```python
from build123d import *

# Parameters (mm, degrees)
SKETCH1_W           = 38
SKETCH1_H           = 70
BOSS_EXTRUDE1_DEPTH = 5
SKETCH2_R           = 1.5
CUT_EXTRUDE1_DEPTH  = 134.018795664
FILLET1_R           = 3
FILLET2_DEPTH       = 5
SKETCH3_W           = 188
SKETCH3_H           = 3
BOSS_EXTRUDE2_DEPTH = 8
SKETCH4_W           = 5
SKETCH4_H           = 39
BOSS_EXTRUDE3_DEPTH = 8
BOSS_EXTRUDE4_DEPTH = 5
FILLET3_SIZE        = 40
FILLET3_SIZE_2      = 10
FILLET4_SIZE        = 40
FILLET4_SIZE_2      = 10
CUT_EXTRUDE2_DEPTH  = 134.165310942


with BuildPart() as part:
    # Sketch1 → Boss-Extrude1 (new body)
    with BuildSketch(Plane.XY):
        with Locations((19, -35)):
            Rectangle(SKETCH1_W, SKETCH1_H)
        Polygon((-75, 15), (-75, 0), (0, 0), (38, 0), (113, 0), (113, 15), align=None)
    extrude(amount=BOSS_EXTRUDE1_DEPTH)

    # Sketch2 → Cut-Extrude1 (cut, through all)
    with BuildSketch(Plane.XY.offset(5)):
        with Locations((34, -66)):
            Circle(SKETCH2_R)
        with Locations((4, -66)):
            Circle(SKETCH2_R)
        with Locations((4, -40)):
            Circle(SKETCH2_R)
        with Locations((34, -40)):
            Circle(SKETCH2_R)
    extrude(amount=-CUT_EXTRUDE1_DEPTH, mode=Mode.SUBTRACT)

    # Fillet1
    fillet1_edges = [part.edges().sort_by_distance(p)[0] for p in [
        (38, -70, 2.5),
        (0, -70, 2.5),
    ]]
    fillet(fillet1_edges, radius=FILLET1_R)

    # Fillet2: read off the stored shape, not the designer's step
    # Fillet2 outline → Fillet2 (add)
    with BuildSketch(Plane.XY):
        with BuildLine():
            add(Edge.make_bspline(
                [(58, 0), (38, 0), (38, -20)],
                knots=[0, 0, 0, 1, 1, 1], degree=2, weights=[1, 0.052631579, 1]))
            Line((58, 0), (38, 0))
            Line((38, 0), (38, -20))
        make_face()
        with BuildLine():
            Line((0, 0), (-20, 0))
            add(Edge.make_bspline(
                [(-20, 0), (0, 0), (0, -20)],
                knots=[0, 0, 0, 1, 1, 1], degree=2, weights=[1, 0.052631579, 1]))
            Line((0, -20), (0, 0))
        make_face()
    extrude(amount=FILLET2_DEPTH)

    # Sketch3 → Boss-Extrude2 (add)
    with BuildSketch(Plane.XY.offset(5)):
        with Locations((19, 4.5)):
            Rectangle(SKETCH3_W, SKETCH3_H)
    extrude(amount=BOSS_EXTRUDE2_DEPTH)

    # Sketch4 → Boss-Extrude3 (add)
    with BuildSketch(Plane.XY.offset(5)):
        with Locations((19, -16.5)):
            Rectangle(SKETCH4_W, SKETCH4_H)
    extrude(amount=BOSS_EXTRUDE3_DEPTH)

    # Sketch5 → Boss-Extrude4 (add)
    with BuildSketch(Plane.XY.offset(5)):
        Polygon((-52, 0), (-57.902965871, 0), (-60, 0), (0, -30), (0, -25), align=None)
        Polygon((38, -30), (98, 0), (90, 0), (38, -25), align=None)
    extrude(amount=-BOSS_EXTRUDE4_DEPTH)

    # Fillet3
    # a fillet whose section is not a circle: 40, 10 mm, written as the material it takes off along each edge
    with BuildSketch(Plane(origin=(-75, 15, -100), x_dir=(1, 0, 0), z_dir=(0, 0, 1))) as fillet3_piece_1:
        with BuildLine():
            Bezier((FILLET3_SIZE, 0), (0, 0), (0, -FILLET3_SIZE_2), weights=[1, 0.707106781, 1])
            Line((0, -FILLET3_SIZE_2), (0, 0))
            Line((0, 0), (FILLET3_SIZE, 0))
        make_face()
    extrude(amount=205, mode=Mode.SUBTRACT)

    # Fillet4
    # a fillet whose section is not a circle: 40, 10 mm, written as the material it takes off along each edge
    with BuildSketch(Plane(origin=(113, 15, -100), x_dir=(-1, 0, 0), z_dir=(0, 0, 1))) as fillet4_piece_1:
        with BuildLine():
            Bezier((FILLET4_SIZE, 0), (0, 0), (0, FILLET4_SIZE_2), weights=[1, 0.707106781, 1])
            Line((0, FILLET4_SIZE_2), (0, 0))
            Line((0, 0), (FILLET4_SIZE, 0))
        make_face()
    extrude(amount=205, mode=Mode.SUBTRACT)

    # Sketch6 → Cut-Extrude2 (cut, through all)
    with BuildSketch(Plane.XY.offset(5)):
        with BuildLine():
            Line((3.671572875, -13.862410437), (-3.399494937, -6.791342626))
            ThreePointArc((-3.399494937, -6.791342626), (-3.399494937, -1.134488376), (2.257359313, -1.134488376))
            Line((2.257359313, -1.134488376), (9.328427125, -8.205556188))
            ThreePointArc((9.328427125, -8.205556188), (9.328427125, -13.862410437), (3.671572875, -13.862410437))
        make_face()
        with BuildLine():
            Line((28.671572875, -8.445013015), (35.742640687, -1.373945203))
            ThreePointArc((35.742640687, -1.373945203), (41.399494937, -1.373945203), (41.399494937, -7.030799453))
            Line((41.399494937, -7.030799453), (34.328427125, -14.101867265))
            ThreePointArc((34.328427125, -14.101867265), (28.671572875, -14.101867265), (28.671572875, -8.445013015))
        make_face()
    extrude(amount=-CUT_EXTRUDE2_DEPTH, mode=Mode.SUBTRACT)


solid = part.part
```
Verification items for the finished model (mm, model axes). A direction names the side the tool comes from. Give positions to 0.01 mm unless a question says otherwise; leave off trailing zeros. Order: outer loops, then holes, each group sorted by start corner. A loop starts at its lowest first (then second) coordinate and runs counter-clockwise, first axis right, second up. Notation, with made-up numbers: (4, -35.5) -> (44, -35.5) arc R27 ccw to (44, -18.5) -> close; hole circle Ø3 at (77.5, -38.75). An arc over 180 degrees is marked (long way). Use a Markdown table: item, result.
1) Material ranges on probe 1 along X at (y, z) = (-66, 3.15); probe 2 along Y at (x, z) = (34, 2.3); probe 3 along X at (y, z) = (-18.5, 3.5), recorded low to high.
Results:
| item | result |
|---|---|
| probe 1 | 0 to 2.5, 5.5 to 32.5, 35.5 to 38 |
| probe 2 | -70 to -67.5, -64.5 to -41.5, -38.5 to -14.4, -3.12 to 15 |
| probe 3 | -23 to -13.52, -1.04 to 39.04, 51.52 to 61 |
2) Depth check by flat-ended pin: pin 1 Ø4 at (y, z) = (-20.5, 9) entering from -X; pin 2 Ø1.5 at (y, z) = (-22, 1.5) entering from +X; pin 3 Ø2 at (y, z) = (-13.5, 4.5) entering from -X; pin 4 Ø1.8 at (x, y) = (4, -40) entering from +Z. Enter the tip coordinate at first touch or a pass-through.
Results:
| item | result |
|---|---|
| pin 1 | x = 16.5 |
| pin 2 | x = 55.5 |
| pin 3 | x = -35 |
| pin 4 | through |
3) Section check C-C, the plane y = -11.5. Give the number of separate pieces and of enclosed holes in the cut face, then the cut area to 3 significant figures.
Results:
| item | result |
|---|---|
| separate pieces | 5 |
| enclosed holes | 0 |
| area | 301 mm² |
4) Section check B-B, the plane x = 13.5. Record the boundary of the cut face in (y, z).
Results:
| item | result |
|---|---|
| outline | (-70, 0) -> (15, 0) -> (15, 5) -> (6, 5) -> (6, 13) -> (3, 13) -> (3, 5) -> (-70, 5) -> close |
5) Tool access check on faces 1 (the flat face through (105, 0, 2)), 2 (the flat face through (-30, 3, 9)), 3 (the flat face through (0.19, -10.38, 2.54)), 4 (the flat face through (21.5, -17, 9)). Record the directions out of +Z, -Z, +X, -X, +Y, -Y that give a thin tool (end or side, any length) a straight path to the whole face; none if there is none.
Results:
| item | result |
|---|---|
| face 1 | +Z, -Z, +X, -Y |
| face 2 | +Z, -X, -Y |
| face 3 | +Z, -Z |
| face 4 | +Z, +X, -Y |
6) Section check A-A, the plane x = -31. Record the boundary of the cut face in (y, z).
Results:
| item | result |
|---|---|
| outline | (-14.5, 0) -> (-10.1, 0) -> (-10.1, 5) -> (-14.5, 5) -> close; (0, 0) -> (15, 0) -> (15, 5) -> (6, 5) -> (6, 13) -> (3, 13) -> (3, 5) -> (0, 5) -> close |
7) Mould release check, pull along X, two halves, no side actions. Record for faces 5 (the flat face through (38, -49, 2)), 6 (the flat face through (32.158, -4.959, 2.535)), 7 (the flat face through (19, -36, 9)): pulls with the +X half, pulls with the -X half, needs draft (parallel to the pull), parting line crosses it, or undercut.
Results:
| item | result |
|---|---|
| face 5 | pulls with the +X half |
| face 6 | undercut |
| face 7 | needs draft |
